Answer from the drawing. Dimensions are ordinates in mm from the lowest x, y and z of the part. A direction names the side the tool comes from. Give positions to 0.01 mm unless a question says otherwise; leave off trailing zeros. Order: outer loops, then holes, each group sorted by start corner. A loop starts at its lowest first (then second) coordinate and runs counter-clockwise, first axis right, second up.
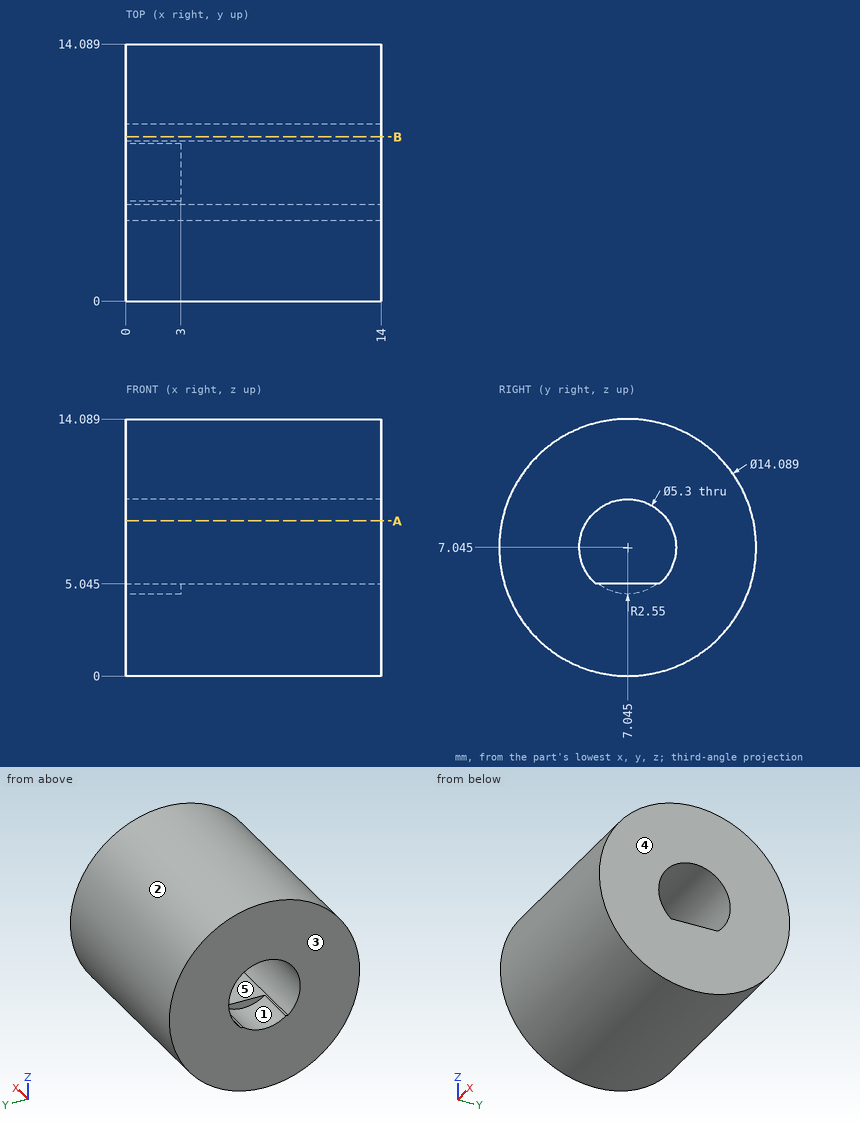
1. Straight lines are drawn through the part: probe 1 along Y at (x, z) = (2, 7) (1 decimal); probe 2 along Y at (x, z) = (13, 6); probe 3 along Z at (x, y) = (9.25, 7.75) (1 decimal). For each, find the intervals that lie inside material, in ascending order.
Findings below:
probe 1: y = 0 to 4.4, 9.7 to 14.1
probe 2: y = 0.08 to 4.61, 9.48 to 14.01
probe 3: z = 0 to 5, 9.6 to 14.1
2. The part is cut by section A-A (z = 8.5). Write down the section's boundary in (x, y).
Findings below:
outline: (0, 0.15) - (14, 0.15) - (14, 4.83) - (0, 4.83) - close; (0, 9.26) - (14, 9.26) - (14, 13.94) - (0, 13.94) - close
3. Which of the six approach directions +Z, -Z, +X, -X, +Y, -Y give full straight-line access (tool end or side, diameter ignored) to the marked faces 4 and 5?
Findings below:
face 4: +Z, -Z, +X, +Y, -Y
face 5: +X, -X
4. The part is cut by section B-B (y = 9). Write down the section's boundary in (x, z), then the cut area to 3 significant figures.
Findings below:
outline: (0, 0.28) - (14, 0.28) - (14, 5.26) - (0, 5.26) - close; (0, 8.83) - (14, 8.83) - (14, 13.81) - (0, 13.81) - close
area: 139 mm2
5. The mould has two halves that part along Y. Classify the marked faces 1, 2 and 3: pulls with the +Y half, pulls with the -Y half, needs draft (parallel to the pull), parting line crosses it, or undercut.
Findings below:
face 1: undercut
face 2: parting line crosses it
face 3: needs draft
